CAD build for the part. Positions are in the model's coordinates, mm. A direction names the side the tool comes from. Give positions to 0.01 mm unless a question says otherwise; leave off trailing zeros. Loops run counter-clockwise (first coordinate to the right, second up) from the corner with the lowest first, then second, coordinate; pieces in that order, holes last.
```python
from build123d import *

# Parameters (mm, degrees)
PAD_DEPTH    = 7
SKETCH001_R  = 1.75
POCKET_DEPTH = 5


with BuildPart() as part:
    # Sketch → Pad (new body)
    with BuildSketch(Plane.XY):
        with BuildLine():
            ThreePointArc((-95.967531, 2.496613), (-95.991882, 1.248412), (-96, 0))
            Line((-100, 0), (-96, 0))
            ThreePointArc((-99.96883, 2.496613), (-99.992207, 1.248404), (-100, 0))
            Line((-99.96883, 2.496613), (-95.967531, 2.496613))
        make_face()
    extrude(amount=PAD_DEPTH)

    # Sketch001 (on Face1 of Pad) → Pocket (cut)
    with BuildSketch(Plane(origin=(0, 2.496613, 0), x_dir=(-1, 0, 0), z_dir=(0, 1, 0))):
        with Locations((97, 3.5)):
            Circle(SKETCH001_R)
    extrude(amount=-POCKET_DEPTH, mode=Mode.SUBTRACT)


solid = part.part
```
1. Saw through at A-A, the plane x = -97. List the corners of the cut face in (y, z), and give its area (3 significant figures).
Responses:
outline: (0, 0) - (2.5, 0) - (2.5, 1.75) - (0, 1.75) - close; (0, 5.25) - (2.5, 5.25) - (2.5, 7) - (0, 7) - close
area: 8.74 mm2
2. Saw through at B-B, the plane y = 1.9. List the corners of the cut face in (x, z), and give its area (3 significant figures).
Responses:
outline: (-99.98, 0) - (-95.98, 0) - (-95.98, 2.08) arc R1.75 cw (long way) to (-95.98, 4.92) - (-95.98, 7) - (-99.98, 7) - close
area: 19.8 mm2
3. Tool access for faces 1 (the face through (-95.99, 1.27, 5.94)), 2 (the face through (-99.99, 1.27, 3.45)), 3 (the face through (-98, 1, 7)): list every direction of +Z, -Z, +X, -X, +Y, -Y with a clear straight run to the whole face (end or side of a thin tool).
Responses:
face 1: +Z, -Z, +X, -Y
face 2: +Z, -Z, -X, +Y
face 3: +Z, +X, -X, +Y, -Y
4. Saw through at C-C, the plane z = 3.5. List the corners of the cut face in (x, y).
Responses:
outline: (-100, 0) - (-98.75, 0) - (-98.75, 2.5) - (-99.97, 2.5) arc R100 ccw to start
5. Drop flat-ended pins along their axis: pin 1 (1 mm diameter, centred on y = 0.5, z = 2.5, fed in from +X); pin 2 (2 mm diameter, centred on x = -97, z = 3.5, fed in from +Y). Give the stop position or say it passes through.
Responses:
pin 1: stops at x = -96
pin 2: passes through
6. Probe line 1 along Z through (x, y) = (-97, 1.35); line 2 along Z through (x, y) = (-97.7, 0.8); line 3 along X through (y, z) = (0.6, 3.5). List the from-to ranges inside material, lowest first.
Responses:
line 1: z = 0 to 1.75, 5.25 to 7
line 2: z = 0 to 1.9, 5.1 to 7
line 3: x = -100 to -98.75
7. Pull direction X, two halves, no side cores. Call faces 4 (the face through (-99, 0, 3)), 5 (the face through (-98.75, 1.27, 3.45)), 6 (the face through (-95.99, 1.27, 1.03)): released by +X, released by -X, zero draft, split by the parting line, or undercut.
Responses:
face 4: zero draft
face 5: undercut
face 6: released by +X
